Geometry check sheet. Reference: the model listing, model coordinates, mm. A direction names the side the tool comes from. Give positions to 0.01 mm unless a question says otherwise; leave off trailing zeros. Order: outer loops, then holes, each group sorted by start corner. A loop starts at its lowest first (then second) coordinate and runs counter-clockwise, first axis right, second up. Notation, with made-up numbers: M -2,37 L 49,37 A19 ccw 49,55 Z; hole C 83,-4 d2. An arc over 180 degrees is marked long. Answer as CSV lines item,"result". Start each with the question number.
Q1. Thickness scan on line 1 (Z direction, x = -29, y = 7); line 2 (Y direction, x = -9, z = 60); line 3 (Y direction, x = -23, z = 65.5). Record the ranges inside material, lowest first.
Q2. Section check A-A, the plane y = -16.5. Record the boundary of the cut face in (x, z).
Q3. Section check C-C, the plane z = 55. Record the boundary of the cut face in (x, y).
Q4. Set-up check for faces 1 (the cylindrical face through (-7.65, -17.46, 71.14)), 2 (the cylindrical face through (27.035, -32.148, 3.042)): record each of +Z, -Z, +X, -X, +Y, -Y from which the full face is reachable in a straight line by a thin tool's end or side.
Q5. Section check D-D, the plane y = 11.5. Record the boundary of the cut face in (x, z) (1 decimal), then the cut area to 3 significant figures.
Q6. Go/stop test with flat-tipped pins: pin 1 (1.5 mm diameter, centred on x = -22.5, y = -6, fed in from +Z); pin 2 (5 mm diameter, centred on y = -9.5, z = 40.5, fed in from +X); pin 3 (12 mm diameter, centred on y = -22, z = 30.5, fed in from +X); pin 4 (4 mm diameter, centred on x = -21.46, y = -5, fed in from -Z). Record where each tip stops, or that it passes through.
Q7. Mould release check, pull along Y, two halves, no side actions. Record for faces 3 (the flat face through (30.042, -5, 3)), 4 (the flat face through (-21, -5, 61)), 5 (the flat face through (-10, 25, 3)): +Y half, -Y half, draft (parallel to the pull), parting line (faces both ways), or undercut.
Q8. Section check B-B, the plane x = -26.5. Record the boundary of the cut face in (y, z), then the cut area to 3 significant figures.
```python
from build123d import *

# Parameters (mm, degrees)
SKETCH_1_W          = 80
SKETCH_1_H          = 60
EXTRUDE_1_DEPTH     = 6
SKETCH_2_R          = 20
EXTRUDE_2_DEPTH     = 75
SKETCH_7_R          = 2.5
CUT_EXTRUDE_2_DEPTH = 20
FILLET_1_R          = 10
CUT_REVOLVE_1_ANGLE = 180


with BuildPart() as part:
    # 草图1 → 凸台-拉伸1 (new body)
    with BuildSketch(Plane.XY):
        with Locations((-9.9578316, -5)):
            Rectangle(SKETCH_1_W, SKETCH_1_H)
    extrude(amount=EXTRUDE_1_DEPTH)

    # 草图2 → 凸台-拉伸2 (add)
    with BuildSketch(Plane.XY.offset(6)):
        with Locations((-9.9578316, -5)):
            Circle(SKETCH_2_R)
    extrude(amount=EXTRUDE_2_DEPTH)

    # 草图7 → 切除-拉伸2 (cut)
    with BuildSketch(Plane.XY.offset(81)):
        with Locations((-9.9578316, -16.5)):
            Circle(SKETCH_7_R)
        with Locations((-21.4578316, -5)):
            Circle(SKETCH_7_R)
        with Locations((1.5421684, -5)):
            Circle(SKETCH_7_R)
    extrude(amount=-CUT_EXTRUDE_2_DEPTH, mode=Mode.SUBTRACT)

    # 圆角1
    fillet_1_edges = [part.edges().sort_by_distance(p)[0] for p in [
        (30.0421684, -35, 3),
        (-49.9578316, -35, 3),
        (-49.9578316, 25, 3),
        (30.0421684, 25, 3),
    ]]
    fillet(fillet_1_edges, radius=FILLET_1_R)

    # 草图4 → 切除-旋转1 (revolve, cut)
    with BuildSketch(Plane.XY.offset(81)):
        with BuildLine():
            Line((-9.9578316, -2), (-9.9578316, 18))
            ThreePointArc((-9.9578316, 18), (0.0421684, 8), (-9.9578316, -2))
        make_face()
    revolve(axis=Axis((-9.9578316, -2, 81), (0, 1, 0)), revolution_arc=CUT_REVOLVE_1_ANGLE, mode=Mode.SUBTRACT)


solid = part.part
```
Answer block:
1,line 1,"z = 0 to 6"
1,line 2,"y = -24.98 to 14.98"
1,line 3,"y = -20.16 to -6.97, -3.03 to 10.16"
2,outline,"M -49.96,0 L 30.04,0 L 30.04,6 L 6.41,6 L 6.41,81 L -7.46,81 L -7.46,61 L -12.46,61 L -12.46,81 L -26.32,81 L -26.32,6 L -49.96,6 Z"
3,outline,"C -9.96,-5 d40"
4,face 1,"+Z"
4,face 2,"+Z, -Z, +X, -Y"
5,outline,"M -50,0 L 30,0 L 30,6 L 1.3,6 L 1.3,81 L -0.6,81 A9.4 cw -19.3,81 L -21.3,81 L -21.3,6 L -50,6 Z"
5,area,"2,040 mm2"
6,pin 1,"stops at z = 61"
6,pin 2,"stops at x = 9.94"
6,pin 3,"stops at x = 6.75"
6,pin 4,"stops at z = 0"
7,face 3,"draft"
7,face 4,"undercut"
7,face 5,"+Y half"
8,outline,"M -35,0 L 25,0 L 25,6 L 6.24,6 L 6.24,81 L -16.24,81 L -16.24,6 L -35,6 Z"
8,area,"2,050 mm2"
